Autodesk Inventor part; units mm, degrees
ref_plane "YZ Plane" through (0, 0, 0) normal (1, 0, 0) x (0, 1, 0)
ref_plane "XZ Plane" through (0, 0, 0) normal (0, 1, 0) x (-1, 0, 0)
ref_plane "XY Plane" through (0, 0, 0) normal (0, 0, 1) x (1, 0, 0)
sketch "Sketch1" plane through (0, 0, 0) normal (0, 0, 1) x (1, 0, 0)
  line L0 (-7.4374, 26) -> (-7, 31)
  line L1 (0, 31) -> (0, 0) construction
  line L2 (-7, 31) -> (0, 31)
  line L3 (-9.5, 26) -> (-9.5, 24.9337)
  line L4 (-12.5, 26) -> (-12.5, 24.9337)
  line L5 (-7.4374, 26) -> (-9.5, 26)
  line L6 (-12.5, 26) -> (-22.6771, 26)
  arc A0 (-12.5, 24.9337) -> (-9.5, 24.9337) centre (-11, 23.5) ccw
  line L7 (-22.6771, -26) -> (-16, -26)
  line L8 (0, -23) -> (0, 0) construction
  arc A1 (-26, -22.6771) -> (-22.6771, -26) centre (0, 0) ccw
  arc A2 (-22.6771, 26) -> (-26, 22.6771) centre (0, 0) ccw
  line L9 (-26, 16) -> (-23, 13)
  line L10 (-23, -13) -> (-26, -16)
  line L11 (-26, 22.6771) -> (-26, 16)
  line L12 (-26, -16) -> (-26, -22.6771)
  line L13 (-16, -26) -> (-13, -23)
  line L14 (-23, 4) -> (-26, 4)
  line L15 (-26, 4) -> (-26, 2)
  line L16 (-26, 2) -> (-25, 2)
  line L17 (-25, 2) -> (-25, 3)
  line L18 (-25, 3) -> (-23, 3)
  line L19 (-23, -4) -> (-26, -4)
  line L20 (-26, -4) -> (-26, -2)
  line L21 (-26, -2) -> (-25, -2)
  line L22 (-25, -2) -> (-25, -3)
  line L23 (-25, -3) -> (-23, -3)
  line L24 (-4, -23) -> (-4, -26)
  line L25 (-4, -26) -> (-2, -26)
  line L26 (-2, -26) -> (-2, -25)
  line L27 (-2, -25) -> (-3, -25)
  line L28 (-3, -25) -> (-3, -23)
  line L29 (-23, 13) -> (-23, 4)
  line L30 (-23, 3) -> (-23, -3)
  line L31 (-23, -4) -> (-23, -13)
  line L32 (-13, -23) -> (-4, -23)
  line L33 (-3, -23) -> (0, -23)
  arc A3 (0, 20.5) -> (0, -20.5) centre (0, 0) ccw
  line L34 (0, 36.125) -> (0, -43.6282) construction
  line L35 (7.4374, 26) -> (7, 31)
  line L36 (7, 31) -> (0, 31)
  line L37 (9.5, 26) -> (9.5, 24.9337)
  line L38 (12.5, 26) -> (12.5, 24.9337)
  line L39 (7.4374, 26) -> (9.5, 26)
  line L40 (12.5, 26) -> (22.6771, 26)
  arc A4 (9.5, 24.9337) -> (12.5, 24.9337) centre (11, 23.5) ccw
  line L41 (22.6771, -26) -> (16, -26)
  arc A5 (22.6771, -26) -> (26, -22.6771) centre (0, 0) ccw
  arc A6 (26, 22.6771) -> (22.6771, 26) centre (0, 0) ccw
  line L42 (26, 16) -> (23, 13)
  line L43 (23, -13) -> (26, -16)
  line L44 (26, 22.6771) -> (26, 16)
  line L45 (26, -16) -> (26, -22.6771)
  line L46 (16, -26) -> (13, -23)
  line L47 (23, 4) -> (26, 4)
  line L48 (26, 4) -> (26, 2)
  line L49 (26, 2) -> (25, 2)
  line L50 (25, 2) -> (25, 3)
  line L51 (25, 3) -> (23, 3)
  line L52 (23, -4) -> (26, -4)
  line L53 (26, -4) -> (26, -2)
  line L54 (26, -2) -> (25, -2)
  line L55 (25, -2) -> (25, -3)
  line L56 (25, -3) -> (23, -3)
  line L57 (4, -23) -> (4, -26)
  line L58 (4, -26) -> (2, -26)
  line L59 (2, -26) -> (2, -25)
  line L60 (2, -25) -> (3, -25)
  line L61 (3, -25) -> (3, -23)
  line L62 (23, 13) -> (23, 4)
  line L63 (23, 3) -> (23, -3)
  line L64 (23, -4) -> (23, -13)
  line L65 (13, -23) -> (4, -23)
  line L66 (3, -23) -> (0, -23)
  arc A7 (0, -20.5) -> (0, 20.5) centre (0, 0) ccw
  point P0 (-20, 20)
  point P1 (-20, -20)
  point P2 (20, 20)
  point P3 (20, -20)
  dimension "d3" = 7.4374
  dimension "d4" = 7
  dimension "d6" = 31
  dimension "d7" = 5
  dimension "d8" = 3
  dimension "d9" = 2.075
  dimension "d10" = 2.5
  dimension "d11" = 11
  dimension "d15" = 34.5
  dimension "d16" = 34.5
  dimension "d19" = 26
  dimension "d20" = 13
  dimension "d21" = 26
  dimension "d22" = 26
  dimension "d23" = 6.6771
  dimension "d24" = 23
  dimension "d25" = 1
  dimension "d26" = 1
  dimension "d27" = 26
  dimension "d28" = 8
  dimension "d29" = 4
  dimension "d30" = 4
  dimension "d31" = 2
  dimension "d32" = 20.5
  dimension "d33" = 40
  dimension "d34" = 20
  dimension "d35" = 20
extrude "SMC, 40MM" add sketch "Sketch1" along normal blind 25.4
hole "Hole1" at (-20, 20, 0) at (-20, -20, 0) at (20, 20, 0) at (20, -20, 0) direction (0, 0, 1) diameter 5.1054 end through all
equation "\"d20\" = 0.5 * d19"
equation "\"d26\" = d25"
equation "\"d30\" = 0.5 * d28"
properties part number "EXTRUSION, CYLINDER, ALUMINIUM, SMC, 40MM" material "Extrusion, Aluminum, SMC, 40 MM"
CAD build for the part. Positions are in the model's coordinates, mm. A direction names the side the tool comes from. Give positions to 0.01 mm unless a question says otherwise; leave off trailing zeros. Write each loop counter-clockwise with the first axis right and the second up, starting at its lowest first coordinate (ties: lowest second). Pieces come first, ordered by that corner, then holes. Notation, with made-up numbers: M 34.25,-16 L 78.25,-16 A20 cw 78.25,6 Z; hole C -9,8 d7. An arc over 180 degrees is marked long. Put each result on its own line as item: value. Start each with the question number.
(1) Flat gauge pins, fed straight in: pin 1 Ø8 at (x, z) = (11.5, 7.5) entering from +Y; pin 2 Ø4 at (y, z) = (-7.5, 19.5) entering from +X; pin 3 Ø1 at (y, z) = (-24.5, 12.5) entering from -X. Where does each tip first touch, or does it go through?
(2) Band-saw the part on D-D, the plane y = 23.5. Write the cut outline in (x, z), and give its area (3 significant figures).
(3) Which spindle directions (+Z, -Z, +X, -X, +Y, -Y) get a long thin tool onto all of the face, cutting with end or side? Do faces 1 (the face through (-24, 4, 13)), 2 (the face through (-23, 0, 13)), 3 (the face through (-9, -23, 13)), 4 (the face through (24, -4, 13)), 5 (the face through (-18, 26, 13)). Say none if no direction does.
(4) Probe L1, parallel to Y at x = -18.5, z = 2.5; L2, parallel to Y at x = 21, z = 11; L3, parallel to X at y = 0, z = 7.5. List the from-to ranges inside material, lowest first.
(5) Band-saw the part on A-A, the plane x = 0. Write the cut outline in (y, z), and give its area (3 significant figures).
(6) Mould opens along X. For faces 6 (the face through (17.848, 21.372, 12.878)), 7 (the face through (-8, 26, 13)), 8 (the face through (-26, -19, 13)) say: +X half, -X half, draft (parallel to the pull), parting line (faces both ways), or undercut.
(7) Band-saw the part on B-B, the plane y = 0. Write the cut outline in (x, z), and give its area (3 significant figures).
(8) Band-saw the part on C-C, the plane x = 19. Write the cut outline in (y, z).
Response values:
1. pin 1: stops at y = 26
1. pin 2: stops at x = 23
1. pin 3: stops at x = -24.78
2. outline: M -25.26,0 L -13.07,0 L -13.07,25.4 L -25.26,25.4 Z; M -8.93,0 L 8.93,0 L 8.93,25.4 L -8.93,25.4 Z; M 13.07,0 L 25.26,0 L 25.26,25.4 L 13.07,25.4 Z
2. area: 1,070 mm2
3. face 1: +Z, -Z, -X
3. face 2: +Z, -Z
3. face 3: +Z, -Z, -Y
3. face 4: +Z, -Z, +X
3. face 5: +Z, -Z, -X, +Y
4. L1: y = -26 to -22.07, -17.93 to -8.83, 8.83 to 17.93, 22.07 to 26
4. L2: y = -26 to -22.35, -17.65 to 17.65, 22.35 to 26
4. L3: x = -23 to -20.5, 20.5 to 23
5. outline: M -23,0 L -20.5,0 L -20.5,25.4 L -23,25.4 Z; M 20.5,0 L 31,0 L 31,25.4 L 20.5,25.4 Z
5. area: 330 mm2
6. face 6: undercut
6. face 7: draft
6. face 8: -X half
7. outline: M -23,0 L -20.5,0 L -20.5,25.4 L -23,25.4 Z; M 20.5,0 L 23,0 L 23,25.4 L 20.5,25.4 Z
7. area: 127 mm2
8. outline: M -26,0 L -22.35,0 L -22.35,25.4 L -26,25.4 Z; M -17.65,0 L -7.7,0 L -7.7,25.4 L -17.65,25.4 Z; M 7.7,0 L 17.65,0 L 17.65,25.4 L 7.7,25.4 Z; M 22.35,0 L 26,0 L 26,25.4 L 22.35,25.4 Z
